```python
from build123d import *

# Parameters (mm, degrees)
ESQUISSE2_W             = 64
ESQUISSE2_H             = 50
ESQUISSE2_R             = 11.5
ESQUISSE2_R_2           = 4
ESQUISSE2_R_3           = 2
ESQUISSE2_R_4           = 1.8
ESQUISSE2_W_2           = 7
ESQUISSE2_H_2           = 9.3
BOSS_EXTRU_1_DEPTH      = 3
BOSS_EXTRU_2_DEPTH      = 6
ENL_V_MAT_EXTRU_1_DEPTH = 6
CHANFREIN1_SIZE         = 4


with BuildPart() as part:
    # Esquisse2 → Boss.-Extru.1 (new, symmetric)
    with BuildSketch(Plane(origin=(0, 0, 0), x_dir=(1, 0, 0), z_dir=(0, 1, 0))):
        Rectangle(ESQUISSE2_W, ESQUISSE2_H)
        with Locations((0, 5)):
            Circle(ESQUISSE2_R, mode=Mode.SUBTRACT)
        with Locations((-18, 5)):
            Circle(ESQUISSE2_R_2, mode=Mode.SUBTRACT)
        with Locations((15.5, -10.5)):
            Circle(ESQUISSE2_R_3, mode=Mode.SUBTRACT)
        with Locations((15.5, 20.5)):
            Circle(ESQUISSE2_R_3, mode=Mode.SUBTRACT)
        with Locations((-15.5, 20.5)):
            Circle(ESQUISSE2_R_3, mode=Mode.SUBTRACT)
        with Locations((-15.5, -10.5)):
            Circle(ESQUISSE2_R_3, mode=Mode.SUBTRACT)
        with Locations((26, 0)):
            Circle(ESQUISSE2_R_4, mode=Mode.SUBTRACT)
        with Locations((-26, 0)):
            Circle(ESQUISSE2_R_4, mode=Mode.SUBTRACT)
        with Locations((26, 11.65)):
            Rectangle(ESQUISSE2_W_2, ESQUISSE2_H_2, mode=Mode.SUBTRACT)
        with Locations((26, -11.65)):
            Rectangle(ESQUISSE2_W_2, ESQUISSE2_H_2, mode=Mode.SUBTRACT)
        with Locations((-26, -11.65)):
            Rectangle(ESQUISSE2_W_2, ESQUISSE2_H_2, mode=Mode.SUBTRACT)
        with Locations((-26, 11.65)):
            Rectangle(ESQUISSE2_W_2, ESQUISSE2_H_2, mode=Mode.SUBTRACT)
    extrude(amount=BOSS_EXTRU_1_DEPTH, both=True)

    # Esquisse3 → Boss.-Extru.2 (add)
    with BuildSketch(Plane(origin=(0, 3, 0), x_dir=(1, 0, 0), z_dir=(0, 1, 0))):
        with BuildLine():
            Line((-7.5, -30), (-7.5, -25))
            Line((-7.5, -25), (-15.5, -25))
            Line((-15.5, -25), (-15.5, -30))
            ThreePointArc((-15.5, -30), (-15.207106781, -30.707106781), (-14.5, -31))
            Line((-14.5, -31), (-8.5, -31))
            ThreePointArc((-8.5, -31), (-7.792893219, -30.707106781), (-7.5, -30))
        make_face()
        with BuildLine():
            Line((15.5, -30), (15.5, -25))
            Line((15.5, -25), (7.5, -25))
            Line((7.5, -25), (7.5, -30))
            ThreePointArc((7.5, -30), (7.792893219, -30.707106781), (8.5, -31))
            Line((8.5, -31), (14.5, -31))
            ThreePointArc((14.5, -31), (15.207106781, -30.707106781), (15.5, -30))
        make_face()
    extrude(amount=-BOSS_EXTRU_2_DEPTH)

    # Esquisse3<3> → Enl_v. mat.-Extru.1 (cut)
    with BuildSketch(Plane(origin=(0, 3, 0), x_dir=(1, 0, 0), z_dir=(0, 1, 0))):
        Polygon((-2.5, -25), (2.5, -25), (2.5, -20), (4.3, -20), (4.3, -14.5), (2.5, -14.5), (2.5, -10.5), (-2.5, -10.5), (-2.5, -14.5), (-4.3, -14.5), (-4.3, -20), (-2.5, -20), align=None)
    extrude(amount=-ENL_V_MAT_EXTRU_1_DEPTH, mode=Mode.SUBTRACT)

    # Chanfrein1
    chanfrein1_edges = [part.edges().sort_by_distance(p)[0] for p in [
        (-32, 0, -25),
    ]]
    chamfer(chanfrein1_edges, length=CHANFREIN1_SIZE)


solid = part.part
```
Verification items for the finished model (mm, model axes). A direction names the side the tool comes from. Round coordinates to 2 decimals unless told otherwise and drop trailing zeros. Write each loop counter-clockwise with the first axis right and the second up, starting at its lowest first coordinate (ties: lowest second). Pieces come first, ordered by that corner, then holes. Notation, with made-up numbers: (24.5, 49.5) - (67.5, 49.5) arc R22 cw to (67.5, 86.5) - close; hole circle Ø10 at (-2.75, 71.5). An arc over 180 degrees is marked (long way). Answer as a JSON object with one key per item and string values. Group by question number.
Q1. Thickness scan on line 1 (Z direction, x = -24, y = 2.25); line 2 (X direction, y = -2.5, z = 7.5); line 3 (X direction, y = -0.5, z = -20.5). Record the ranges inside material, lowest first.
Q2. Go/stop test with flat-tipped pins: pin 1 Ø4.5 at (x, z) = (15.5, 10.5) entering from -Y; pin 2 Ø2.5 at (x, y) = (-0.5, -1) entering from +Z; pin 3 Ø1.4 at (x, y) = (-4, -1) entering from +Z; pin 4 Ø1.5 at (y, z) = (-1, 27) entering from -X. Record where each tip stops, or that it passes through.
Q3. Tool access check on faces 4 (the flat face through (-30, 0, -23)), 5 (the flat face through (-26, 0, 16.3)), 6 (the flat face through (2.5, 0, 13)). Record the directions out of +Z, -Z, +X, -X, +Y, -Y that give a thin tool (end or side, any length) a straight path to the whole face; none if there is none.
Q4. Section check C-C, the plane x = 3.5. Enter the section's corners in (y, z).
Q5. Section check B-B, the plane x = -26. Enter the section's corners in (y, z), plus the area to 3 significant figures.
Q6. Section check A-A, the plane z = 13.5. Enter the section's corners in (x, y).
Q7. Section check D-D, the plane y = -0.75. Give the number of separate pieces and of enclosed holes in the cut face, plus the area to 3 significant figures.
Q8. Mould release check, pull along Z, two halves, no side actions. Record for faces 1 (the flat face through (15.5, 0, 28)), 2 (the flat face through (-5, 0, 25)), 3 (the cylindrical face through (-9.126, -0.042, 1.998)): released by +Z, released by -Z, zero draft, split by the parting line, or undercut.
Found:
{
 "1": {"line 1": "z = -25 to -16.3, -7 to 7, 16.3 to 25", "line 2": "x = -32 to -29.5, -22.5 to 22.5, 29.5 to 32", "line 3": "x = -32 to -17.5, -13.5 to 13.5, 17.5 to 32"},
 "2": {"pin 1": "stops at y = -3", "pin 2": "stops at z = 10.5", "pin 3": "stops at z = 25", "pin 4": "stops at x = -15.5"},
 "3": {"face 4": "-Z, -X, +Y, -Y", "face 5": "+Y, -Y", "face 6": "+Z, +Y, -Y"},
 "4": {"outline": "(-3, -25) - (3, -25) - (3, -15.95) - (-3, -15.95) - close; (-3, 5.95) - (3, 5.95) - (3, 14.5) - (-3, 14.5) - close; (-3, 20) - (3, 20) - (3, 25) - (-3, 25) - close"},
 "5": {"outline": "(-3, -25) - (3, -25) - (3, -16.3) - (-3, -16.3) - close; (-3, -7) - (3, -7) - (3, -1.8) - (-3, -1.8) - close; (-3, 1.8) - (3, 1.8) - (3, 7) - (-3, 7) - close; (-3, 16.3) - (3, 16.3) - (3, 25) - (-3, 25) - close", "area": "167 mm^2"},
 "6": {"outline": "(-32, -3) - (-29.5, -3) - (-29.5, 3) - (-32, 3) - close; (-22.5, -3) - (-2.5, -3) - (-2.5, 3) - (-22.5, 3) - close; (2.5, -3) - (22.5, -3) - (22.5, 3) - (2.5, 3) - close; (29.5, -3) - (32, -3) - (32, 3) - (29.5, 3) - close"},
 "7": {"separate pieces": "1", "enclosed holes": "12", "area": "2,400 mm^2"},
 "8": {"face 1": "zero draft", "face 2": "released by +Z", "face 3": "undercut"}
}
